Model file for the job. Use its own axes, mm. Face numbers are marked on the shaded views. A direction names the side the tool comes from. Coordinates: 2 decimals unless noted, no trailing zeros. Order: outer loops, then holes, each group sorted by start corner. A loop starts at its lowest first (then second) coordinate and runs counter-clockwise, first axis right, second up. Notation, with made-up numbers: (61.5, -26.75) -> (104.5, -26.75) arc R18 ccw to (104.5, 7.25) -> close; hole circle Ø7 at (52.5, 5.5). An arc over 180 degrees is marked (long way). Return JSON: item names as keys, results as strings. Group by question number.
1) Cut at A-A (y = 11). Write the cut outline in (x, z).
2) Flat gauge pins, fed straight in: pin 1 (4 mm diameter, centred on x = 30.5, y = 40.5, fed in from -Z); pin 2 (1 mm diameter, centred on x = 36, z = 16, fed in from -Y); pin 3 (18 mm diameter, centred on x = 26, z = 42, fed in from +Y). Where does each tip first touch, or does it go through?
3) Cut at C-C (z = 41.5). Write the cut outline in (x, y), and give its area (3 significant figures).
4) Pull direction Z, two halves, no side cores. Call the marked faces 1, 2, 3 and 4: +Z half, -Z half, draft (parallel to the pull), parting line (faces both ways), or undercut.
5) Which spindle directions (+Z, -Z, +X, -X, +Y, -Y) get a long thin tool onto all of the face, cutting with end or side? Do the marked faces 5, 6, 7 and 8. Say none if no direction does.
6) Cut at D-D (y = 20). Write the cut outline in (x, z).
7) Probe line 1 (Z direction, x = 15.5, y = 12.5); line 2 (Z direction, x = 13, y = 38); line 3 (Z direction, x = 20, y = 10.5). List the from-to ranges inside material, lowest first.
8) Cut at B-B (x = 13.5). Write the cut outline in (y, z).
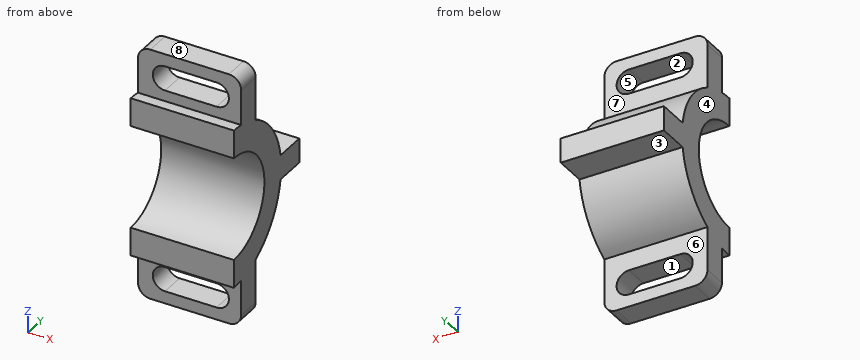
Autodesk Inventor part; units mm, degrees
ref_plane "YZ Plane" through (0, 0, 0) normal (1, 0, 0) x (0, 1, 0)
ref_plane "XZ Plane" through (0, 0, 0) normal (0, 1, 0) x (-1, 0, 0)
ref_plane "XY Plane" through (0, 0, 0) normal (0, 0, 1) x (1, 0, 0)
sketch "草圖1" plane through (0, 0, 0) normal (1, 0, 0) x (0, 1, 0)
  arc A0 (0, -21) -> (0, 21) centre (0, 0) ccw
  line L0 (0, 33.7624) -> (0, -28.793) construction
  line L1 (0, -21) -> (0, -32.5)
  line L2 (15, -28.8314) -> (15, -51.5)
  line L3 (5, -51.5) -> (5, -32.1131)
  arc A1 (0, -32.5) -> (5, -32.1131) centre (0, 0) ccw
  line L4 (5, -51.5) -> (15, -51.5)
  line L5 (0, 0) -> (31.6672, 0)
  line L6 (45, -5) -> (32.1131, -5)
  line L7 (45, -5) -> (45, 0)
  arc A2 (15, -28.8314) -> (32.1131, -5) centre (0, 0) ccw
  line L8 (45, 5) -> (32.1131, 5)
  line L9 (45, 5) -> (45, 0)
  line L10 (15, 28.8314) -> (15, 51.5)
  line L11 (5, 51.5) -> (5, 32.1131)
  line L12 (5, 51.5) -> (15, 51.5)
  arc A3 (32.1131, 5) -> (15, 28.8314) centre (0, 0) ccw
  arc A4 (5, 32.1131) -> (0, 32.5) centre (0, 0) ccw
  line L13 (0, 32.5) -> (0, 21)
  dimension "d0" = 10
  dimension "d2" = 45
  dimension "d4" = 10
  dimension "d6" = 42
  dimension "d7" = 65
  dimension "d9" = 103
  dimension "d10" = 5
extrude "擠出1" add sketch "草圖1" along normal blind 42
fillet "圓角1" radius 5 4 edges at (42, 10, 51.5) (0, 10, 51.5) (42, 10, -51.5) (0, 10, -51.5)
sketch "草圖2" plane through (0, 15, 28.8314) normal (0, 1, 0) x (1, 0, 0)
  arc A0 (11, -7.6686) -> (11, -17.6686) centre (11, -12.6686) ccw
  arc A1 (32, -17.6686) -> (32, -7.6686) centre (32, -12.6686) ccw
  line L0 (32, -7.6686) -> (11, -7.6686)
  line L1 (11, -17.6686) -> (32, -17.6686)
  line L2 (42, 0) -> (42, -17.6686)
  line L3 (0, 28.8314) -> (45.6948, 28.8314)
  arc A2 (11, 75.3314) -> (11, 65.3314) centre (11, 70.3314) ccw
  arc A3 (32, 65.3314) -> (32, 75.3314) centre (32, 70.3314) ccw
  line L4 (32, 65.3314) -> (11, 65.3314)
  line L5 (11, 75.3314) -> (32, 75.3314)
  line L6 (5, -22.6686) -> (37, -22.6686)
  point P0 (42, 75.3314)
  dimension "d14" = 10
  dimension "d15" = 21
  dimension "d16" = 10
  dimension "d17" = 83
extrude "擠出2" cut sketch "草圖2" against normal blind 42
properties part number "練習一"
Answers below:
{
 "1": {"outline": "(0, -46.5) arc R5 ccw to (5, -51.5) -> (37, -51.5) arc R5 ccw to (42, -46.5) -> (42, -17.89) -> (0, -17.89) -> close; (0, 17.89) -> (42, 17.89) -> (42, 46.5) arc R5 ccw to (37, 51.5) -> (5, 51.5) arc R5 ccw to (0, 46.5) -> close; hole (11, -46.5) -> (32, -46.5) arc R5 ccw to (32, -36.5) -> (11, -36.5) arc R5 ccw to start; hole (11, 36.5) -> (32, 36.5) arc R5 ccw to (32, 46.5) -> (11, 46.5) arc R5 ccw to start"},
 "2": {"pin 1": "stops at z = -5", "pin 2": "stops at y = 12.99", "pin 3": "stops at y = 15"},
 "3": {"outline": "(0, 5) -> (6, 5) -> (6, 15) -> (0, 15) -> close; (37, 5) -> (42, 5) -> (42, 15) -> (37, 15) -> close", "area": "110 mm^2"},
 "4": {"face 1": "undercut", "face 2": "undercut", "face 3": "-Z half", "face 4": "draft"},
 "5": {"face 5": "+Y, -Y", "face 6": "-Z, +X, -X, +Y", "face 7": "+Z, +X, -X, +Y", "face 8": "+Z, +X, -X, +Y, -Y"},
 "6": {"outline": "(0, -25.62) -> (42, -25.62) -> (42, -6.4) -> (0, -6.4) -> close; (0, 6.4) -> (42, 6.4) -> (42, 25.62) -> (0, 25.62) -> close"},
 "7": {"line 1": "z = -51.5 to -46.5, -36.5 to -16.87, 16.87 to 36.5, 46.5 to 51.5", "line 2": "z = -5 to 5", "line 3": "z = -51.5 to -46.5, -36.5 to -18.19, 18.19 to 36.5, 46.5 to 51.5"},
 "8": {"outline": "(0, -32.5) arc R32.5 ccw to (5, -32.11) -> (5, -36.5) -> (15, -36.5) -> (15, -28.83) arc R32.5 ccw to (32.11, -5) -> (45, -5) -> (45, 5) -> (32.11, 5) arc R32.5 ccw to (15, 28.83) -> (15, 36.5) -> (5, 36.5) -> (5, 32.11) arc R32.5 ccw to (0, 32.5) -> (0, 21) arc R21 cw to (0, -21) -> close; (5, -51.5) -> (15, -51.5) -> (15, -46.5) -> (5, -46.5) -> close; (5, 46.5) -> (15, 46.5) -> (15, 51.5) -> (5, 51.5) -> close"}
}
